```python
from build123d import *

# Parameters (mm, degrees)
SKETCH1_W                  = 177.8
SKETCH1_H                  = 76.2
MILLING_SUPPORT_BASE_DEPTH = 19.05
BOLT_SLOT_LEFT_END_DEPTH   = 20.05
BOLT_SLOT_RIGHT_END_DEPTH  = 20.05
OUTER_TRIANGLE_DEPTH       = 9.525
INNER_TRIANGLE_DEPTH       = 48.625
FILLET_AT_TRIANGLE_BASE_R  = 3.81


with BuildPart() as part:
    # Sketch1 → Milling Support Base (new body)
    with BuildSketch(Plane(origin=(0, 0, 0), x_dir=(1, 0, 0), z_dir=(0, 1, 0))):
        with Locations((12.7, 0)):
            Rectangle(SKETCH1_W, SKETCH1_H)
    extrude(amount=-MILLING_SUPPORT_BASE_DEPTH)

    # Sketch2 → Bolt Slot Left End (cut, through all)
    with BuildSketch(Plane(origin=(0, 0, 0), x_dir=(1, 0, 0), z_dir=(0, 1, 0))):
        with BuildLine():
            Line((-76.2, 6.35), (-57.15, 6.35))
            ThreePointArc((-57.15, 6.35), (-50.8, 0), (-57.15, -6.35))
            Line((-57.15, -6.35), (-76.2, -6.35))
            Line((-76.2, -6.35), (-76.2, 6.35))
        make_face()
    extrude(amount=-BOLT_SLOT_LEFT_END_DEPTH, mode=Mode.SUBTRACT)

    # Sketch3 → Bolt Slot Right End (cut, through all)
    with BuildSketch(Plane.XZ.offset(19.05)):
        with BuildLine():
            Line((101.6, 6.35), (82.55, 6.35))
            ThreePointArc((82.55, 6.35), (76.2, 0), (82.55, -6.35))
            Line((82.55, -6.35), (101.6, -6.35))
            Line((101.6, -6.35), (101.6, 6.35))
        make_face()
    extrude(amount=-BOLT_SLOT_RIGHT_END_DEPTH, mode=Mode.SUBTRACT)

    # Sketch4 → Outer Triangle (add, symmetric)
    with BuildSketch(Plane.XY):
        Polygon((-36.408550143, 0), (-36.408550143, 152.4), (-11.008550143, 152.4), (64.959238023, 25.4), (64.959238023, 0), align=None)
    extrude(amount=OUTER_TRIANGLE_DEPTH, both=True)

    # Sketch5 → Inner Triangle (cut, through all)
    with BuildSketch(Plane.XY.offset(9.525)):
        with BuildLine():
            Line((-4.658550143, 31.75), (20.365749185, 31.75))
            ThreePointArc((20.365749185, 31.75), (25.889412512, 34.967645701), (25.81522023, 41.359718598))
            Line((25.81522023, 41.359718598), (0.790920902, 83.194371039))
            ThreePointArc((0.790920902, 83.194371039), (-6.349460972, 86.055381202), (-11.008550143, 79.934652441))
            Line((-11.008550143, 79.934652441), (-11.008550143, 38.1))
            ThreePointArc((-11.008550143, 38.1), (-9.148678203, 33.609871939), (-4.658550143, 31.75))
        make_face()
    extrude(amount=-INNER_TRIANGLE_DEPTH, mode=Mode.SUBTRACT)

    # Fillet at Triangle base
    fillet_at_triangle_base_edges = [part.edges().sort_by_distance(p)[0] for p in [
        (14.27534394, 0, -9.525),
        (-36.408550143, 0, 0),
        (64.959238023, 0, 0),
        (14.27534394, 0, 9.525),
    ]]
    fillet(fillet_at_triangle_base_edges, radius=FILLET_AT_TRIANGLE_BASE_R)


solid = part.part
```
Part model, mm, in its own coordinate system. A direction names the side the tool comes from. Give positions to 0.01 mm unless a question says otherwise; leave off trailing zeros. Write each loop counter-clockwise with the first axis right and the second up, starting at its lowest first coordinate (ties: lowest second). Pieces come first, ordered by that corner, then holes. Notation, with made-up numbers: (-4, 75) -> (39, 75) arc R10 ccw to (39, 92) -> close; hole circle Ø5 at (34, 74.5). An arc over 180 degrees is marked (long way). Put each result on its own line as item: value. Start each with the question number.
Item 1: Which spindle directions (+Z, -Z, +X, -X, +Y, -Y) get a long thin tool onto all of the face, cutting with end or side? Do faces 5 (the face through (92, -10, -6.35)), 6 (the face through (-36.409, 77, 0)), 7 (the face through (15, 63, -9.525)). Say none if no direction does.
Item 2: Cut at B-B (y = -4). List the corners of the cut face in (x, z), then the cut area to 3 significant figures.
Item 3: Pull direction X, two halves, no side cores. Call faces 1 (the face through (13.48, 61.98, 0.13)), 2 (the face through (-11.009, 59, 0)), 3 (the face through (-76.2, -9, 22)), 4 (the face through (76.2, -9.7, 0.1)): pulls with the +X half, pulls with the -X half, needs draft (parallel to the pull), parting line crosses it, or undercut.
Item 4: Cut at D-D (x = 13). List the corners of the cut face in (y, z) (3 decimals).
Item 5: Pin check, flat tips, straight feed: pin 1 Ø5.5 at (x, z) = (8.5, -0.5) entering from +Y; pin 2 Ø21 at (y, z) = (81.5, -2.5) entering from -X; pin 3 Ø8 at (x, y) = (-44, 94) entering from +Z; pin 4 Ø15 at (y, z) = (12, 3) entering from +X. Stop position of each tip, or through.
Item 6: Cut at C-C (x = -23). List the corners of the cut face in (y, z) (3 decimals).
Item 7: Cut at A-A (z = 0). List the corners of the cut face in (x, y), then the cut area to 3 significant figures.
Item 8: Wall check: L1, parallel to Y at x = 78, z = -10; L2, parallel to Z at x = -9, y = 117 (3 decimals); L3, parallel to Y at x = 67, z = 0. Give the ranges that are in metal, low to high. Write a range as [from, to].
Answer list:
1. face 5: +X, +Y, -Y
1. face 6: +Z, -Z, -X, +Y
1. face 7: -Z, +X, -X, +Y
2. outline: (-76.2, -38.1) -> (101.6, -38.1) -> (101.6, -6.35) -> (82.55, -6.35) arc R6.35 cw to (82.55, 6.35) -> (101.6, 6.35) -> (101.6, 38.1) -> (-76.2, 38.1) -> (-76.2, 6.35) -> (-57.15, 6.35) arc R6.35 cw to (-57.15, -6.35) -> (-76.2, -6.35) -> close
2. area: 12,900 mm2
3. face 1: undercut
3. face 2: undercut
3. face 3: pulls with the -X half
3. face 4: pulls with the +X half
4. outline: (-19.05, -38.1) -> (0, -38.1) -> (0, -13.335) arc R3.81 cw to (3.81, -9.525) -> (31.75, -9.525) -> (31.75, 9.525) -> (3.81, 9.525) arc R3.81 cw to (0, 13.335) -> (0, 38.1) -> (-19.05, 38.1) -> close; (62.784, -9.525) -> (112.263, -9.525) -> (112.263, 9.525) -> (62.784, 9.525) -> close
5. pin 1: stops at y = 124.38
5. pin 2: stops at x = -36.41
5. pin 3: passes through
5. pin 4: stops at x = 64.96
6. outline: (-19.05, -38.1) -> (0, -38.1) -> (0, -13.335) arc R3.81 cw to (3.81, -9.525) -> (152.4, -9.525) -> (152.4, 9.525) -> (3.81, 9.525) arc R3.81 cw to (0, 13.335) -> (0, 38.1) -> (-19.05, 38.1) -> close
7. outline: (-50.8, -19.05) -> (76.2, -19.05) -> (76.2, 0) -> (68.77, 0) arc R3.81 cw to (64.96, 3.81) -> (64.96, 25.4) -> (-11.01, 152.4) -> (-36.41, 152.4) -> (-36.41, 3.81) arc R3.81 cw to (-40.22, 0) -> (-50.8, 0) -> close; hole (-11.01, 38.1) arc R6.35 ccw to (-4.66, 31.75) -> (20.37, 31.75) arc R6.35 ccw to (25.82, 41.36) -> (0.79, 83.19) arc R6.35 ccw to (-11.01, 79.93) -> close
7. area: 11,700 mm2
8. L1: y = [-19.05, 0]
8. L2: z = [-9.525, 9.525]
8. L3: y = [-19.05, 0.44]
